from build123d import *

# Parameters (mm, degrees)
SKETCH1_W           = 22.03
SKETCH1_H           = 25.05
SKETCH1_R           = 1.5
BOSS_EXTRUDE1_DEPTH = 4
SKETCH2_W           = 26.03
SKETCH2_H           = 29.05
SKETCH2_W_2         = 22.03
SKETCH2_H_2         = 25.05
BOSS_EXTRUDE3_DEPTH = 14
CUT_EXTRUDE1_DEPTH  = 5
CUT_EXTRUDE2_DEPTH  = 50
SKETCH5_W           = 4
SKETCH5_H           = 1
CUT_EXTRUDE3_DEPTH  = 50
CUT_EXTRUDE4_DEPTH  = 1


with BuildPart() as part:
    # Sketch1 → Boss-Extrude1 (new body)
    with BuildSketch(Plane(origin=(0, 0, 0), x_dir=(1, 0, 0), z_dir=(0, 1, 0))):
        with Locations((9.515, 11.025)):
            Rectangle(SKETCH1_W, SKETCH1_H)
        with Locations(Location((16.53, 2.5, 0), (0, 0, 270))):
            Circle(SKETCH1_R, mode=Mode.SUBTRACT)
        with Locations(Location((16.53, 19.55, 0), (0, 0, 270))):
            Circle(SKETCH1_R, mode=Mode.SUBTRACT)
    extrude(amount=BOSS_EXTRUDE1_DEPTH)

    # Sketch2 → Boss-Extrude3 (add)
    with BuildSketch(Plane.XZ):
        with Locations((9.515, -11.025)):
            Rectangle(SKETCH2_W, SKETCH2_H)
        with Locations((9.515, -11.025)):
            Rectangle(SKETCH2_W_2, SKETCH2_H_2, mode=Mode.SUBTRACT)
    extrude(amount=-BOSS_EXTRUDE3_DEPTH)

    # Sketch3 → Cut-Extrude1 (cut)
    with BuildSketch(Plane.ZY.offset(3.5)):
        Polygon((-11.025, 4), (-23.025, 4), (-23.025, 7), (0.975, 7), (0.975, 4), align=None)
    extrude(amount=-CUT_EXTRUDE1_DEPTH, mode=Mode.SUBTRACT)

    # Sketch4 → Cut-Extrude2 (cut)
    with BuildSketch(Plane.ZY.offset(3.5)):
        Polygon((-11.025, 14), (-13.025, 14), (-13.025, 13), (-9.025, 13), (-9.025, 14), align=None)
    extrude(amount=-CUT_EXTRUDE2_DEPTH, mode=Mode.SUBTRACT)

    # Sketch5 → Cut-Extrude3 (cut)
    with BuildSketch(Plane(origin=(0, 0, -25.55), x_dir=(-1, 0, 0), z_dir=(0, 0, -1))):
        with Locations((-15.53, 13.5)):
            Rectangle(SKETCH5_W, SKETCH5_H)
    extrude(amount=-CUT_EXTRUDE3_DEPTH, mode=Mode.SUBTRACT)

    # Sketch7 → Cut-Extrude4 (cut)
    with BuildSketch(Plane.XZ):
        Polygon((-3.5, -11.025), (-3.5, -6.275), (22.53, -6.275), (22.53, -15.775), (-3.5, -15.775), align=None)
    extrude(amount=-CUT_EXTRUDE4_DEPTH, mode=Mode.SUBTRACT)


solid = part.part
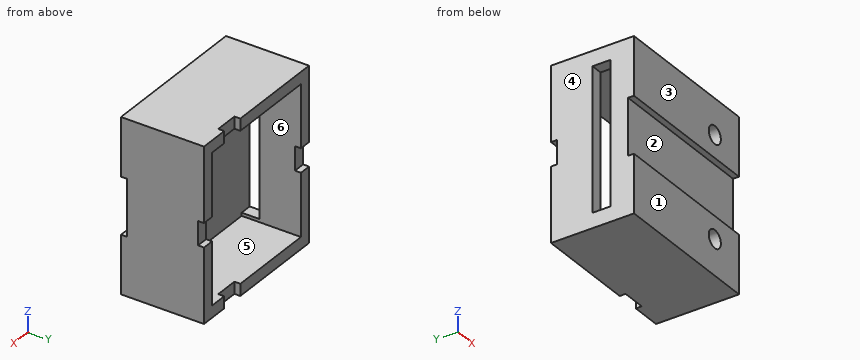
Can you work these out from the model? Positions are in its coordinate system, mm. Face numbers are marked on the shaded views. A direction names the side the tool comes from. Coordinates: 2 decimals unless noted, no trailing zeros. Write each loop counter-clockwise with the first axis right and the second up, starting at its lowest first coordinate (ties: lowest second). Pieces come first, ordered by that corner, then holes. Notation, with made-up numbers: (-9.75, 56.25) -> (3.25, 56.25) arc R15 cw to (3.25, 60.25) -> close; hole circle Ø4 at (-17, 53.5). An arc over 180 degrees is marked (long way). Answer as CSV lines item,"result".
1) On a 3-axis mill with a long thin cutter (end or side, diameter ignored), from which of +Z, -Z, +X, -X, +Y, -Y can I reach the whole of each face in a straight line? I mean the marked faces 1 and 2. Say none if no direction works.
Check result:
face 1,"+Z, -Z, +X, -X, -Y"
face 2,"+X, -X, -Y"
2) If we section it at B-B on z = -6.75: Please give me the cut outline in (x, y).
Check result:
outline,"(-3.5, 1) -> (22.53, 1) -> (22.53, 14) -> (20.53, 14) -> (20.53, 4) -> (-3.5, 4) -> close; (-3.5, 7) -> (-1.5, 7) -> (-1.5, 14) -> (-3.5, 14) -> close"
3) If I drill on line 1 (X direction, y = 12.75, z = -4); line 2 (X direction, y = 3.2, z = -19.55); line 3 (Z direction, x = 0.5, y = 9.25), over which ranges is the centre line in solid material (lowest first)? Write a range as from..to.
Check result:
line 1,"-3.5..-1.5, 20.53..22.53"
line 2,"-3.5..15.03, 18.03..22.53"
line 3,"-25.55..-23.55, 1.5..3.5"
4) If we mould it in two halves opening along X, with no side actions, what happens to the marked faces 3, 4, 5 and 6? For each: +X half, -X half, draft (parallel to the pull), parting line (faces both ways), or undercut.
Check result:
face 3,"draft"
face 4,"-X half"
face 5,"undercut"
face 6,"undercut"
5) If we section it at D-D on x = 8: Please give me the cut outline in (y, z) (3 decimals), then the cut area to 3 significant figures.
Check result:
outline,"(0, -25.55) -> (14, -25.55) -> (14, -23.55) -> (4, -23.55) -> (4, 1.5) -> (14, 1.5) -> (14, 3.5) -> (0, 3.5) -> (0, -6.275) -> (1, -6.275) -> (1, -15.775) -> (0, -15.775) -> close"
area,"147 mm²"
6) Will these pins go through, and if not, where does the flat tip stop? P1, Ø6, axis at x = 13, z = -10.5, coming from the -Y side; P2, Ø6, axis at x = -1, z = -19, coming from the -Y side; P3, Ø10, axis at x = 11, z = -5.5, coming from the +Y side.
Check result:
P1,"y = 1"
P2,"y = 0"
P3,"y = 4"
7) If we section it at C-C on y = 3: Please give me the cut outline in (x, z), then the cut area to 3 significant figures.
Check result:
outline,"(-3.5, -25.55) -> (22.53, -25.55) -> (22.53, 3.5) -> (-3.5, 3.5) -> close; hole circle Ø3 at (16.53, -19.55); hole circle Ø3 at (16.53, -2.5)"
area,"742 mm²"
8) If we section it at A-A on z = -19.55: Please give me the cut outline in (x, y).
Check result:
outline,"(-3.5, 0) -> (15.03, 0) -> (15.03, 4) -> (-3.5, 4) -> close; (-3.5, 7) -> (-1.5, 7) -> (-1.5, 14) -> (-3.5, 14) -> close; (18.03, 0) -> (22.53, 0) -> (22.53, 14) -> (20.53, 14) -> (20.53, 4) -> (18.03, 4) -> close"
